The listing builds one solid part. Answer for the finished solid, in the listing's coordinates (mm). A direction names the side the tool comes from. Coordinates: 2 decimals unless noted, no trailing zeros. Loops run counter-clockwise (first coordinate to the right, second up) from the corner with the lowest first, then second, coordinate; pieces in that order, holes last. Notation, with made-up numbers: (35, 74.5) - (51, 74.5) arc R15 cw to (51, 100.5) - close; hole circle Ø6 at (32, 24.25). An arc over 180 degrees is marked (long way). Return JSON: item names as keys, results as strings. Group by question number.
1. Section B-B (x = 0) is taken. Write down the section's boundary in (y, z), and give its area (3 significant figures).
2. Section C-C (z = 17.5) is taken. Write down the section's boundary in (x, y).
3. Which of the six approach directions +Z, -Z, +X, -X, +Y, -Y give full straight-line access (tool end or side, diameter ignored) to faces 1 (the face through (-6.324, 7.395, 4.032)), 2 (the face through (9, 18, 9)), 3 (the face through (18.765, 16.521, 0.806))?
4. Section A-A (z = 0) is taken. State how many separate pieces and enclosed holes the cut face has, and give its area (3 significant figures).
5. The mould has two halves that part along X. Classify faces 4 (the face through (9, 15, 0)), 5 (the face through (0, 17, 16)), 6 (the face through (6.654, 26.451, 3.461)): pulls with the +X half, pulls with the -X half, needs draft (parallel to the pull), parting line crosses it, or undercut.
6. Section D-D (y = 2) is taken. Write down the section's boundary in (x, z), and give its area (3 significant figures).
7. Find the intervals of material crossed by line 1 along X through (y, z) = (17, 0); line 2 along X through (y, z) = (24, 0); line 3 along Y through (x, z) = (17, 9), in increasing order.
8. Each of these flat-tipped pins is pushed along its axis until it touches: P1, Ø8, axis at y = 13, z = 8.5, coming from the +X side; P2, Ø1.8, axis at x = 0, z = 17.5, coming from the -Y side; P3, Ø1.5, axis at x = 3, y = 11, coming from the -Z side; P4, Ø7, axis at x = 0, z = 0, coming from the +Y side. Where does it stop, or does it pass through?
```python
from build123d import *

# Parameters (mm, degrees)
FILLET1_R               = 5
SKETCH3_R               = 1.5
CUT_EXTRUDE2_DEPTH      = 35.124771062
CUT_EXTRUDE3_DEPTH      = 46.872104813
CUT_EXTRUDE3_DEPTH_BACK = 46.872104813


with BuildPart() as part:
    # Sketch2 → Revolve1 (revolve)
    with BuildSketch(Plane.XY, mode=Mode.PRIVATE) as revolve1_sk:
        Polygon((7.5, 30), (7.5, 18), (20.5, 18), (20.5, 15), (7.5, 15), (7.5, 0), (3, 0), (3, 30), align=None)
    revolve(revolve1_sk.sketch.rotate(Axis((0, 9.767689721, 0), (0, -1, 0)), 90), axis=Axis((0, 9.767689721, 0), (0, -1, 0)))

    # Fillet1
    fillet1_edges = [part.edges().sort_by_distance(p)[0] for p in [
        (0, 18, -7.5),
    ]]
    fillet(fillet1_edges, radius=FILLET1_R)

    # Sketch3 → Cut-Extrude2 (cut, through all)
    with BuildSketch(Plane(origin=(0, 18, 0), x_dir=(1, 0, 0), z_dir=(0, 1, 0))):
        with Locations(Location((0, 17.5, 0), (0, 0, 270))):
            Circle(SKETCH3_R)
        with Locations(Location((17.5, 0, 0), (0, 0, 270))):
            Circle(SKETCH3_R)
        with Locations(Location((0, -17.5, 0), (0, 0, 270))):
            Circle(SKETCH3_R)
        with Locations(Location((-17.5, 0, 0), (0, 0, 270))):
            Circle(SKETCH3_R)
    extrude(amount=-CUT_EXTRUDE2_DEPTH, mode=Mode.SUBTRACT)

    # Sketch4 → Cut-Extrude3 (cut, two sides: drawn at the far end of the back side and taken through both)
    with BuildSketch(Plane.ZY.offset(7.5).offset(-CUT_EXTRUDE3_DEPTH_BACK)):
        with BuildLine():
            ThreePointArc((1.5, 26.5), (0.324875311, 27.964396132), (-1.35927471, 27.134328198))
            Line((-1.35927471, 27.134328198), (1.35927471, 25.865671802))
            ThreePointArc((1.35927471, 25.865671802), (1.464396132, 26.175124689), (1.5, 26.5))
        make_face()
        with BuildLine():
            Line((1.35927471, 25.865671802), (-1.35927471, 27.134328198))
            ThreePointArc((-1.35927471, 27.134328198), (-0.634328198, 25.14072529), (1.35927471, 25.865671802))
        make_face()
    extrude(amount=CUT_EXTRUDE3_DEPTH + CUT_EXTRUDE3_DEPTH_BACK, mode=Mode.SUBTRACT)


solid = part.part
```
The answers:
{
 "1": {"outline": "(0, -7.5) - (15, -7.5) - (15, -16) - (18, -16) - (18, -12.5) arc R5 cw to (23, -7.5) - (30, -7.5) - (30, -3) - (0, -3) - close; (0, 3) - (30, 3) - (30, 7.5) - (23, 7.5) arc R5 cw to (18, 12.5) - (18, 16) - (15, 16) - (15, 7.5) - (0, 7.5) - close; (15, -20.5) - (18, -20.5) - (18, -19) - (15, -19) - close; (15, 19) - (18, 19) - (18, 20.5) - (15, 20.5) - close", "area": "341 mm2"},
 "2": {"outline": "(-10.68, 15) - (-1.5, 15) - (-1.5, 18) - (-10.68, 18) - close; (1.5, 15) - (10.68, 15) - (10.68, 18) - (1.5, 18) - close"},
 "3": {"face 1": "-Y", "face 2": "+Y", "face 3": "+Y, -Y"},
 "4": {"separate pieces": "6", "enclosed holes": "0", "area": "314 mm2"},
 "5": {"face 4": "needs draft", "face 5": "undercut", "face 6": "parting line crosses it"},
 "6": {"outline": "circle Ø15 at (0, 0); hole circle Ø6 at (0, 0)", "area": "148 mm2"},
 "7": {"line 1": "x = -20.5 to -19, -16 to -3, 3 to 16, 19 to 20.5", "line 2": "x = -7.5 to -3, 3 to 7.5", "line 3": "y = 15 to 18"},
 "8": {"P1": "stops at x = 19.87", "P2": "passes through", "P3": "stops at z = -7.15", "P4": "stops at y = 30"}
}
